Read the model definition and answer for the solid it produces. Units are mm, in the model's axes. Round coordinates to 2 decimals unless told otherwise and drop trailing zeros. Write each loop counter-clockwise with the first axis right and the second up, starting at its lowest first coordinate (ties: lowest second). Pieces come first, ordered by that corner, then holes. Notation, with made-up numbers: M 21.25,6 L 43.25,6 A23 ccw 43.25,27 Z; hole C 66.5,-30.75 d6. An arc over 180 degrees is marked long. Use one line per item in the form item = value. Start each with the question number.
```python
from build123d import *

# Parameters (mm, degrees)
SKETCH1_R           = 60
SKETCH1_R_2         = 2.637642313
BOSS_EXTRUDE1_DEPTH = 1


with BuildPart() as part:
    # Sketch1 → Boss-Extrude1 (new body)
    with BuildSketch(Plane(origin=(0, 0, 0), x_dir=(1, 0, 0), z_dir=(0, 1, 0))):
        with BuildLine():
            Line((77.459067431, -74.053128544), (77.459067431, 75.622473214))
            ThreePointArc((77.459067431, 75.622473214), (76.57640363, 77.753412133), (74.445464711, 78.636075934))
            Line((74.445464711, 78.636075934), (-75.230137046, 78.636075934))
            ThreePointArc((-75.230137046, 78.636075934), (-77.361075965, 77.753412133), (-78.243739766, 75.622473214))
            Line((-78.243739766, 75.622473214), (-78.243739766, -74.053128544))
            ThreePointArc((-78.243739766, -74.053128544), (-77.361075965, -76.184067463), (-75.230137046, -77.066731264))
            Line((-75.230137046, -77.066731264), (74.445464711, -77.066731264))
            ThreePointArc((74.445464711, -77.066731264), (76.57640363, -76.184067463), (77.459067431, -74.053128544))
        make_face()
        with Locations((-0.392336167, 0.784672335)):
            Circle(SKETCH1_R, mode=Mode.SUBTRACT)
        with Locations((-60.606097453, -59.429088951)):
            Circle(SKETCH1_R_2, mode=Mode.SUBTRACT)
        with Locations((-60.606097453, 60.998433621)):
            Circle(SKETCH1_R_2, mode=Mode.SUBTRACT)
        with Locations((59.821425118, -59.429088951)):
            Circle(SKETCH1_R_2, mode=Mode.SUBTRACT)
        with Locations((59.821425118, 60.998433621)):
            Circle(SKETCH1_R_2, mode=Mode.SUBTRACT)
    extrude(amount=BOSS_EXTRUDE1_DEPTH)


solid = part.part
```
Q1. Find section C-C on y = 0.85. Write down the section's boundary in (x, z), and give its area (3 significant figures).
Q2. Straight lines are drawn through the part: line 1 (X direction, y = 0.45, z = 60); line 2 (Z direction, x = -1, y = 0.65); line 3 (Z direction, x = 23, y = 0.8). For each, find the intervals that lie inside material, in ascending order. Write a range as [from, to].
Q3. Find section A-A on z = 21. Write down the section's boundary in (x, y).
Q4. Find section B-B on x = -20.5. Write down the section's boundary in (y, z), and give its area (3 significant figures).
Q5. For a pull along X with two mould halves and no side action, classify faces 1 (the face through (-53, 0, -36)), 2 (the face through (-58.17, 0.49, -59.99)) as +X half, -X half, draft (parallel to the pull), parting line (faces both ways), or undercut.
Response:
q1.outline = M -78.24,-75.62 A3.01 ccw -75.23,-78.64 L 74.45,-78.64 A3.01 ccw 77.46,-75.62 L 77.46,74.05 A3.01 ccw 74.45,77.07 L -75.23,77.07 A3.01 ccw -78.24,74.05 Z; hole C -60.61,-61 d5.28; hole C -60.61,59.43 d5.28; hole C -0.39,-0.78 d120; hole C 59.82,-61 d5.28; hole C 59.82,59.43 d5.28
q1.area = 12,800 mm²
q2.line_1 = [-78.24, -63.18], [-58.03, 57.25], [62.4, 77.46]
q2.line_2 = [-78.64, -60.78], [59.21, 77.07]
q2.line_3 = [-78.64, -56.04], [54.47, 77.07]
q3.outline = M -78.24,0 L -56.3,0 L -56.3,1 L -78.24,1 Z; M 55.51,0 L 77.46,0 L 77.46,1 L 55.51,1 Z
q4.outline = M 0,-78.64 L 1,-78.64 L 1,-57.32 L 0,-57.32 Z; M 0,55.75 L 1,55.75 L 1,77.07 L 0,77.07 Z
q4.area = 42.6 mm²
q5.face_1 = draft
q5.face_2 = undercut
